from build123d import *

# Parameters (mm, degrees)
F0_R     = 30
F0_R_2   = 10
F0_R_3   = 21.5
F0_R_4   = 18.75
F0_R_5   = 6.6
F1_DEPTH = 5
F3_DEPTH = 11


with BuildPart() as f1:
    # F0 (on Top) → F1 (new body)
    with BuildSketch(Plane.XY):
        with BuildLine():
            ThreePointArc((18.3030052177, -31), (31.2642622481, -17.8478543831), (36, 0))
            ThreePointArc((36, 0), (31.2978497092, 17.7888898917), (18.4197442455, 30.9307779069))
            ThreePointArc((18.4197442455, 30.9307779069), (9.5522770937, 34.7095664382), (0, 36))
            ThreePointArc((0, 36), (-18.7386337537, 30.7386337537), (-32, 16.4924225025))
            Line((-32, 16.4924225025), (-32, -16.4924225025))
            ThreePointArc((-32, -16.4924225025), (-18.7386337537, -30.7386337537), (0, -36))
            ThreePointArc((0, -36), (9.4868329805, -34.7275107084), (18.3030052177, -31))
        make_face()
        Circle(F0_R, mode=Mode.SUBTRACT)
        with BuildLine():
            ThreePointArc((242, 16.4924225025), (228.7386337537, 30.7386337537), (210, 36))
            ThreePointArc((210, 36), (200.4477229063, 34.7095664382), (191.5802557545, 30.9307779069))
            ThreePointArc((191.5802557545, 30.9307779069), (174.0000639573, -0.0678595955), (191.6969947823, -31))
            ThreePointArc((191.6969947823, -31), (200.5131670195, -34.7275107084), (210, -36))
            ThreePointArc((210, -36), (228.7386337537, -30.7386337537), (242, -16.4924225025))
            Line((242, -16.4924225025), (242, 16.4924225025))
        make_face()
        with Locations((210, 0)):
            Circle(F0_R, mode=Mode.SUBTRACT)
        Circle(F0_R)
        Circle(F0_R_2, mode=Mode.SUBTRACT)
        with Locations((210, 0)):
            Circle(F0_R)
        with Locations((210, 0)):
            Circle(F0_R_3, mode=Mode.SUBTRACT)
        with Locations((210, 0)):
            Circle(F0_R_3)
        with Locations((210, 0)):
            Circle(F0_R_4, mode=Mode.SUBTRACT)
        with BuildLine():
            ThreePointArc((19.6214168703, 36), (23.4046464655, 33.6633706545), (26.9125802938, 30.9307779069))
            Line((26.9125802938, 30.9307779069), (34, 30.9307779069))
            ThreePointArc((34, 30.9307779069), (37, 33.9307779069), (40, 30.9307779069))
            Line((40, 30.9307779069), (45, 30.9307779069))
            Line((45, 30.9307779069), (165, 30.9307779069))
            Line((165, 30.9307779069), (170, 30.9307779069))
            ThreePointArc((170, 30.9307779069), (173, 33.9307779069), (176, 30.9307779069))
            Line((176, 30.9307779069), (183.0874197062, 30.9307779069))
            ThreePointArc((183.0874197062, 30.9307779069), (186.5953535345, 33.6633706545), (190.3785831296, 36))
            Line((190.3785831296, 36), (19.6214168703, 36))
        make_face()
        with BuildLine():
            Line((34, -31), (26.83281573, -31))
            ThreePointArc((26.83281573, -31), (23.361269906, -33.693487032), (19.6214168703, -36))
            Line((19.6214168703, -36), (190.3785831296, -36))
            ThreePointArc((190.3785831296, -36), (186.638730094, -33.693487032), (183.16718427, -31))
            Line((183.16718427, -31), (176, -31))
            ThreePointArc((176, -31), (173, -34), (170, -31))
            Line((170, -31), (165, -31))
            Line((165, -31), (45, -31))
            Line((45, -31), (40, -31))
            ThreePointArc((40, -31), (37, -34), (34, -31))
        make_face()
        with BuildLine():
            Line((37, 27.9307779069), (37, 17.6635217327))
            ThreePointArc((37, 17.6635217327), (39.9874980463, 9.0553851381), (41, 0))
            ThreePointArc((41, 0), (39.9874980463, -9.0553851381), (37, -17.6635217327))
            Line((37, -17.6635217327), (37, -28))
            ThreePointArc((37, -28), (39.1213203436, -28.8786796564), (40, -31))
            Line((40, -31), (45, -31))
            Line((45, -31), (45, 30.9307779069))
            Line((45, 30.9307779069), (40, 30.9307779069))
            ThreePointArc((40, 30.9307779069), (39.1213203436, 28.8094575634), (37, 27.9307779069))
        make_face()
        with BuildLine():
            ThreePointArc((173, -17.6635217327), (169, 0), (173, 17.6635217327))
            Line((173, 17.6635217327), (173, 27.9307779069))
            ThreePointArc((173, 27.9307779069), (170.8786796564, 28.8094575634), (170, 30.9307779069))
            Line((170, 30.9307779069), (165, 30.9307779069))
            Line((165, 30.9307779069), (165, -31))
            Line((165, -31), (170, -31))
            ThreePointArc((170, -31), (170.8786796564, -28.8786796564), (173, -28))
            Line((173, -28), (173, -17.6635217327))
        make_face()
        Circle(F0_R_2)
        Circle(F0_R_5, mode=Mode.SUBTRACT)
        with BuildLine():
            ThreePointArc((18.4197442455, 30.9307779069), (31.2978497092, 17.7888898917), (36, 0))
            ThreePointArc((36, 0), (31.2642622481, -17.8478543831), (18.3030052177, -31))
            Line((18.3030052177, -31), (26.83281573, -31))
            ThreePointArc((26.83281573, -31), (32.6055594055, -24.8571417474), (37, -17.6635217327))
            Line((37, -17.6635217327), (37, 17.6635217327))
            ThreePointArc((37, 17.6635217327), (32.6375474194, 24.815126404), (26.9125802938, 30.9307779069))
            Line((26.9125802938, 30.9307779069), (18.4197442455, 30.9307779069))
        make_face()
        with BuildLine():
            Line((191.5802557545, 30.9307779069), (183.0874197062, 30.9307779069))
            ThreePointArc((183.0874197062, 30.9307779069), (177.3624525806, 24.815126404), (173, 17.6635217327))
            Line((173, 17.6635217327), (173, -17.6635217327))
            ThreePointArc((173, -17.6635217327), (177.3944405945, -24.8571417474), (183.16718427, -31))
            Line((183.16718427, -31), (191.6969947823, -31))
            ThreePointArc((191.6969947823, -31), (174.0000639573, -0.0678595955), (191.5802557545, 30.9307779069))
        make_face()
        with BuildLine():
            ThreePointArc((41, 0), (39.9874980463, 9.0553851381), (37, 17.6635217327))
            Line((37, 17.6635217327), (37, -17.6635217327))
            ThreePointArc((37, -17.6635217327), (39.9874980463, -9.0553851381), (41, 0))
        make_face()
        with BuildLine():
            Line((173, -17.6635217327), (173, 17.6635217327))
            ThreePointArc((173, 17.6635217327), (169, 0), (173, -17.6635217327))
        make_face()
        with BuildLine():
            ThreePointArc((0, 36), (9.5522770937, 34.7095664382), (18.4197442455, 30.9307779069))
            Line((18.4197442455, 30.9307779069), (26.9125802938, 30.9307779069))
            ThreePointArc((26.9125802938, 30.9307779069), (23.4046464655, 33.6633706545), (19.6214168703, 36))
            Line((19.6214168703, 36), (0, 36))
        make_face()
        with BuildLine():
            Line((210, 36), (190.3785831296, 36))
            ThreePointArc((190.3785831296, 36), (186.5953535345, 33.6633706545), (183.0874197062, 30.9307779069))
            Line((183.0874197062, 30.9307779069), (191.5802557545, 30.9307779069))
            ThreePointArc((191.5802557545, 30.9307779069), (200.4477229063, 34.7095664382), (210, 36))
        make_face()
        with BuildLine():
            Line((26.83281573, -31), (18.3030052177, -31))
            ThreePointArc((18.3030052177, -31), (9.4868329805, -34.7275107084), (0, -36))
            Line((0, -36), (19.6214168703, -36))
            ThreePointArc((19.6214168703, -36), (23.361269906, -33.693487032), (26.83281573, -31))
        make_face()
        with BuildLine():
            ThreePointArc((183.16718427, -31), (186.638730094, -33.693487032), (190.3785831296, -36))
            Line((190.3785831296, -36), (210, -36))
            ThreePointArc((210, -36), (200.5131670195, -34.7275107084), (191.6969947823, -31))
            Line((191.6969947823, -31), (183.16718427, -31))
        make_face()
        with BuildLine():
            ThreePointArc((37, -17.6635217327), (32.6055594055, -24.8571417474), (26.83281573, -31))
            Line((26.83281573, -31), (34, -31))
            ThreePointArc((34, -31), (34.8786796564, -28.8786796564), (37, -28))
            Line((37, -28), (37, -17.6635217327))
        make_face()
        with BuildLine():
            Line((176, -31), (183.16718427, -31))
            ThreePointArc((183.16718427, -31), (177.3944405945, -24.8571417474), (173, -17.6635217327))
            Line((173, -17.6635217327), (173, -28))
            ThreePointArc((173, -28), (175.1213203436, -28.8786796564), (176, -31))
        make_face()
        with BuildLine():
            Line((34, 30.9307779069), (26.9125802938, 30.9307779069))
            ThreePointArc((26.9125802938, 30.9307779069), (32.6375474194, 24.815126404), (37, 17.6635217327))
            Line((37, 17.6635217327), (37, 27.9307779069))
            ThreePointArc((37, 27.9307779069), (34.8786796564, 28.8094575634), (34, 30.9307779069))
        make_face()
        with BuildLine():
            ThreePointArc((173, 17.6635217327), (177.3624525806, 24.815126404), (183.0874197062, 30.9307779069))
            Line((183.0874197062, 30.9307779069), (176, 30.9307779069))
            ThreePointArc((176, 30.9307779069), (175.1213203436, 28.8094575634), (173, 27.9307779069))
            Line((173, 27.9307779069), (173, 17.6635217327))
        make_face()
    extrude(amount=F1_DEPTH)

    # F2 (on face) → F3 (join)
    with BuildSketch(Plane.XY.offset(5)):
        with BuildLine():
            ThreePointArc((32.2300370842, 0), (28.249548951, -9.6195118668), (18.6300370842, -13.6))
            Line((18.6300370842, -13.6), (18.6278837067, -16.5999992272))
            ThreePointArc((18.6278837067, -16.5999992272), (30.3708692945, -11.7408322103), (35.2300363114, 0.0021533775))
            Line((35.2300363114, 0.0021533775), (32.2300370842, 0))
        make_face()
        with BuildLine():
            ThreePointArc((1.4010723087, -16.9409777332), (-16.154736314, -5.264086135), (-8.8464426541, 14.5133013966))
            Line((-8.8464426541, 14.5133013966), (-10.5643945811, 16.9784386755))
            ThreePointArc((-10.5643945811, 16.9784386755), (-18.9787357989, -6.2800054738), (1.6467177805, -19.9309038698))
            Line((1.6467177805, -19.9309038698), (1.4010723087, -16.9409777332))
        make_face()
    extrude(amount=F3_DEPTH)


solid = f1.part
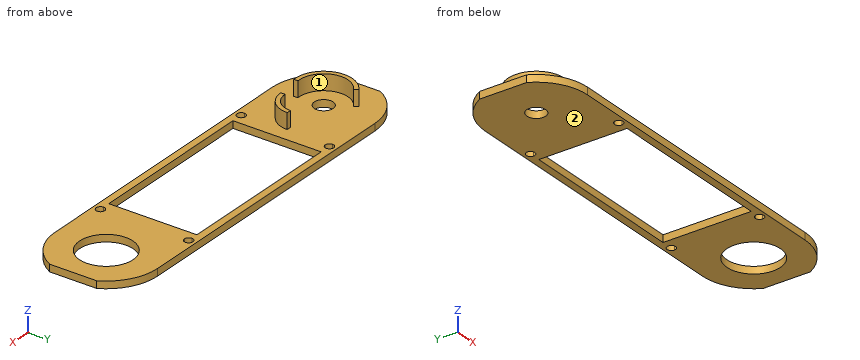
Work out the finished part from the listing and answer in its coordinate system (mm). Face numbers are marked on the shaded views. Round coordinates to 2 decimals unless told otherwise and drop trailing zeros. Loops run counter-clockwise (first coordinate to the right, second up) from the corner with the lowest first, then second, coordinate; pieces in that order, holes last. Notation, with made-up numbers: (54, -11.5) - (98, -11.5) arc R28 cw to (98, 13.5) - close; hole circle Ø7 at (64.25, -17). An arc over 180 degrees is marked (long way). Use one line per item in the form item = value. Start each with the question number.
(1) Find section A-A on z = 11. Determine the outline of the cut face in (x, y), and give its area (3 significant figures).
(2) Flat-ended cylindrical pins translate along their axes: P1, Ø8, axis at x = 0, y = 0, coming from the -Z side (3 decimals); P2, Ø2, axis at y = 6.5, z = 9, coming from the +X side. Find the tip coordinate at first contact, or state that the pin passes through.
(3) Determine the mould class of the marked faces 1 and 2 for opening direction X: +X half, -X half, draft (parallel to the pull), parting line (faces both ways), or undercut.
(4) Find section B-B on y = -10.5. Determine the outline of the cut face in (x, z).
(5) Consider line 1 (Y direction, x = 0, z = 2.35); line 2 (Y direction, x = 68, z = 3.5); line 3 (X direction, y = 32, z = 2). Determine where each line is inside the solid, lowest interval first.
Answer list:
q1.outline = (-10.56, 16.98) arc R20 ccw to (1.65, -19.93) - (1.4, -16.94) arc R17 cw to (-8.85, 14.51) - close; (18.63, -16.6) arc R16.59 ccw to (35.23, 0) - (32.23, 0) arc R13.59 cw to (18.63, -13.6) - close
q1.area = 219 mm^2
q2.P1 = through
q2.P2 = -15.25
q3.face_1 = undercut
q3.face_2 = draft
q4.outline = (-32, 0) - (45, 0) - (45, 5) - (31.49, 5) - (31.49, 16) - (27.28, 16) - (27.28, 5) - (-13.36, 5) - (-13.36, 16) - (-17.01, 16) - (-17.01, 5) - (-32, 5) - close; (165, 0) - (194.47, 0) - (194.47, 5) - (165, 5) - close; (225.53, 0) - (242, 0) - (242, 5) - (225.53, 5) - close
q5.line_1 = -36 to -6.6, 6.6 to 36
q5.line_2 = -36 to -31, 30.93 to 36
q5.line_3 = -16.49 to 34.2, 39.8 to 170.2, 175.8 to 226.49
